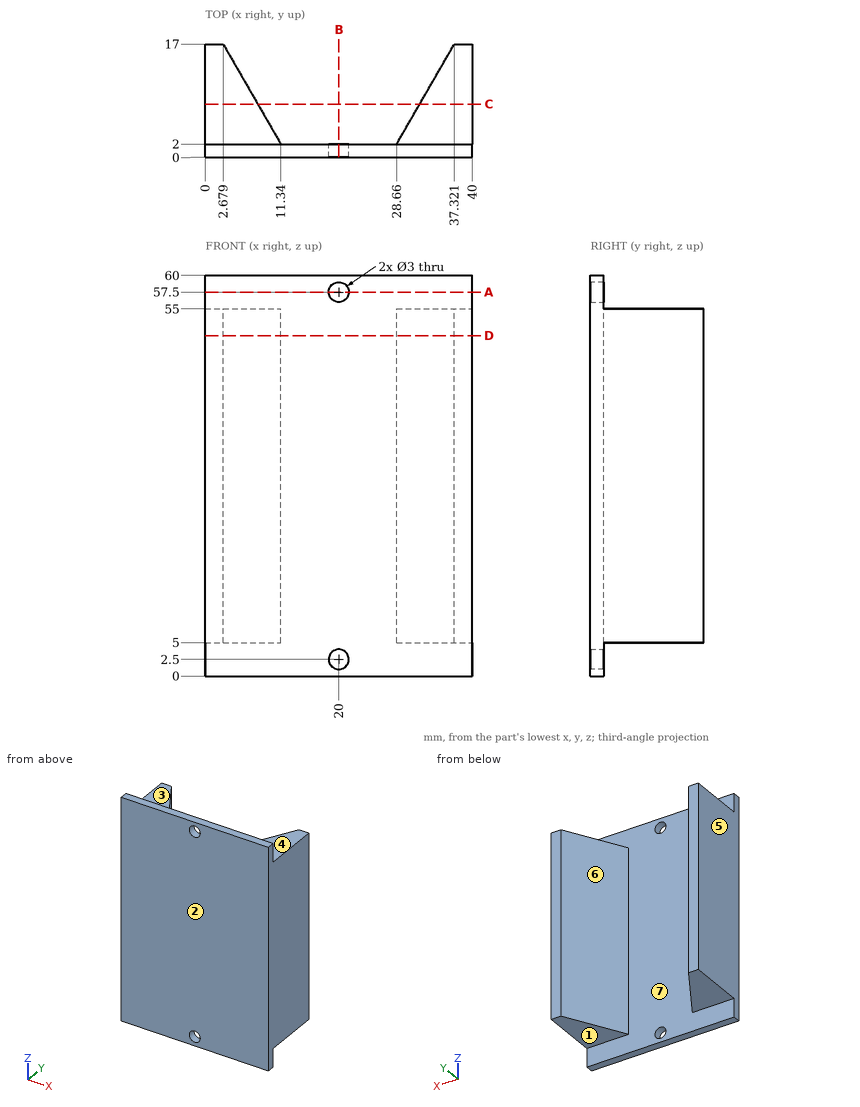
Study the drawing (mm; zero at the part's minimum x, y, z) and answer. A direction names the side the tool comes from. Round coordinates to 2 decimals unless told otherwise and drop trailing zeros. Write each loop counter-clockwise with the first axis right and the second up, starting at its lowest first coordinate (ties: lowest second). Pieces come first, ordered by that corner, then holes. Notation, with made-up numbers: (-20.75, 38.5) -> (17.25, 38.5) arc R19 ccw to (17.25, 52.5) -> close; hole circle Ø4 at (-19.5, 23). An arc over 180 degrees is marked (long way). Use CSV: the item, a comma, the result in double quotes. Start each with the question number.
(1) Section C-C on y = 8 is taken. Give the vertices of the cut face in (x, z) (1 decimal).
(2) Section D-D on z = 51 is taken. Give the vertices of the cut face in (x, y), then the cut area to 3 significant figures.
(3) Consider L1, parallel to X at y = 0.7, z = 2.5; L2, parallel to Y at x = 26.5, z = 48.5; L3, parallel to X at y = 11, z = 8 (1 decimal). Determine where each line is inside the solid, lowest interval first. Write a range as from..to.
(4) The mould has two halves that part along X. Classify the marked faces 4, 5, 6 and 7: released by +X, released by -X, zero draft, split by the parting line, or undercut.
(5) Section B-B on x = 20 is taken. Give the vertices of the cut face in (y, z), then the cut area to 3 significant figures.
(6) Section A-A on z = 57.5 is taken. Give the vertices of the cut face in (x, y).
(7) Each of these flat-tipped pins is pushed along its axis until it touches: pin 1 (3.5 mm diameter, centred on x = 7.5, y = 7.5, fed in from +Z); pin 2 (4 mm diameter, centred on x = 7, y = 10, fed in from -Z); pin 3 (2.5 mm diameter, centred on x = 20, z = 57.5, fed in from -Y); pin 4 (12 mm diameter, centred on x = 16, z = 19, fed in from +Y). Where does it stop, or does it pass through?
(8) Which of the six approach directions +Z, -Z, +X, -X, +Y, -Y give full straight-line access (tool end or side, diameter ignored) to the marked faces 1, 2 and 3?
A:
1,outline,"(0, 5) -> (7.9, 5) -> (7.9, 55) -> (0, 55) -> close; (32.1, 5) -> (40, 5) -> (40, 55) -> (32.1, 55) -> close"
2,outline,"(0, 0) -> (40, 0) -> (40, 17) -> (37.32, 17) -> (28.66, 2) -> (11.34, 2) -> (2.68, 17) -> (0, 17) -> close"
2,area,"290 mm²"
3,L1,"x = 0..18.5, 21.5..40"
3,L2,"y = 0..2"
3,L3,"x = 0..6.1, 33.9..40"
4,face 4,"zero draft"
4,face 5,"released by -X"
4,face 6,"undercut"
4,face 7,"undercut"
5,outline,"(0, 0) -> (2, 0) -> (2, 1) -> (0, 1) -> close; (0, 4) -> (2, 4) -> (2, 56) -> (0, 56) -> close; (0, 59) -> (2, 59) -> (2, 60) -> (0, 60) -> close"
5,area,"108 mm²"
6,outline,"(0, 0) -> (18.5, 0) -> (18.5, 2) -> (0, 2) -> close; (21.5, 0) -> (40, 0) -> (40, 2) -> (21.5, 2) -> close"
7,pin 1,"stops at z = 55"
7,pin 2,"stops at z = 5"
7,pin 3,"passes through"
7,pin 4,"stops at y = 4.32"
8,face 1,"-Z, +X, -X, +Y"
8,face 2,"+Z, -Z, +X, -X, -Y"
8,face 3,"+Z, +X, -X, +Y"
